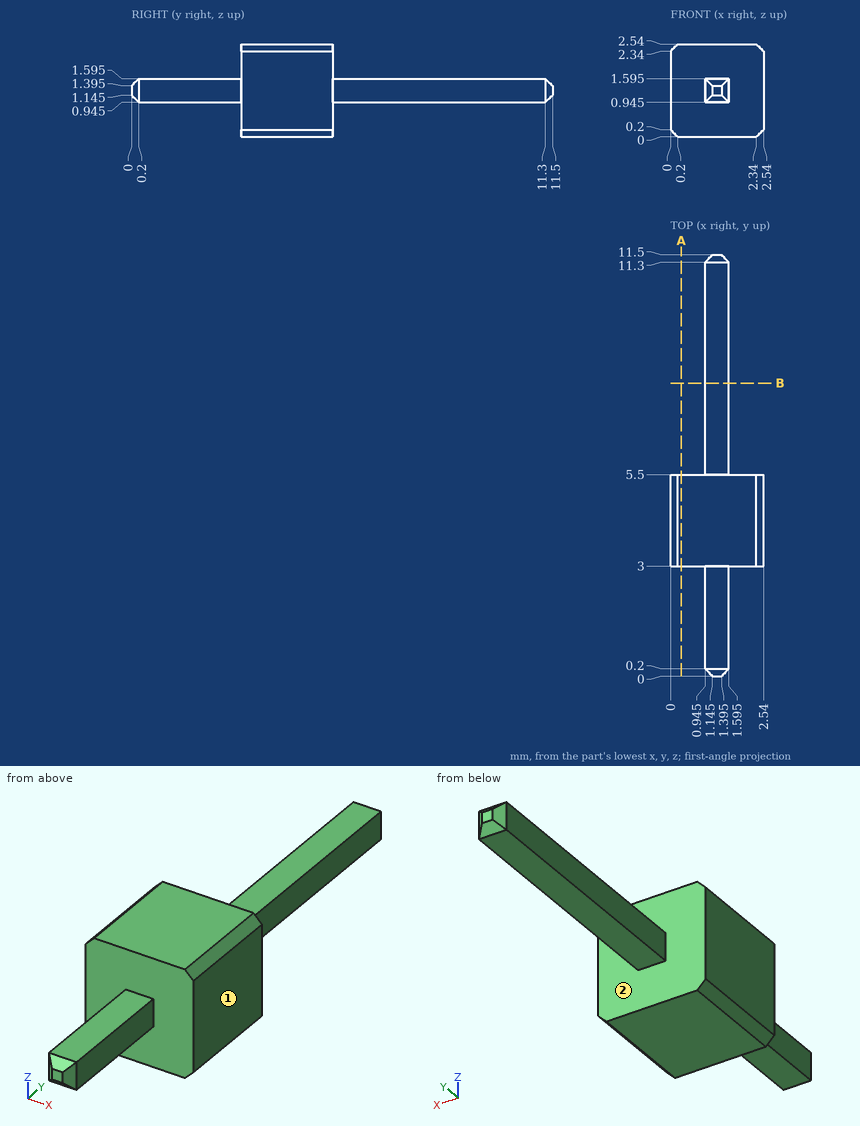
Design review of the part shown in the three views and the two pictorial views. Dimensions are in mm from the part's minimum x, y and z. A direction names the side the tool comes from. Give positions to 0.01 mm unless a question says otherwise; leave off trailing zeros. Write each loop counter-clockwise with the first axis right and the second up, starting at its lowest first coordinate (ties: lowest second). Pieces come first, ordered by that corner, then holes. Notation, with made-up numbers: M -38,-36 L 20,-36 A21 ccw 20,-17 Z; hole C -37.5,39 d2. An arc over 180 degrees is marked long. Answer in a Markdown table with one row per item.
Item 1: Add section A-A on x = 0.3. Give the boundary of the cut face in (y, z).
Check sheet entries:
| item | result |
|---|---|
| outline | M 3,0 L 5.5,0 L 5.5,2.54 L 3,2.54 Z |
Item 2: Tool access review of the marked faces 1 and 2: name each direction out of +Z, -Z, +X, -X, +Y, -Y from which nothing blocks a thin tool from reaching the whole face with its end or side.
Check sheet entries:
| item | result |
|---|---|
| face 1 | +Z, -Z, +X, +Y, -Y |
| face 2 | +Y |
Item 3: For line 1 along Z through (x, y) = (1.55, 2.25) (3 decimals); line 2 along Y through (x, z) = (0.8, 1.6), list the stretches that pass through material, from the lowest coordinate up.
Check sheet entries:
| item | result |
|---|---|
| line 1 | 0.945 to 1.595 |
| line 2 | 3 to 5.5 |
Item 4: For P1, Ø0.5, axis at y = 2, z = 1, coming from the +X side (3 decimals); P2, Ø0.7, axis at x = 1, y = 2, coming from the -Z side (3 decimals); P3, Ø1, axis at x = 1, y = 7, coming from the +Z side (3 decimals), all flat-tipped, find the tip position at first contact; note any pin that passes through.
Check sheet entries:
| item | result |
|---|---|
| P1 | x = 1.595 |
| P2 | z = 0.945 |
| P3 | z = 1.595 |
Item 5: Add section B-B on y = 8. Give the boundary of the cut face in (x, z) (3 decimals).
Check sheet entries:
| item | result |
|---|---|
| outline | M 0.945,0.945 L 1.595,0.945 L 1.595,1.595 L 0.945,1.595 Z |
